Part model, mm, in its own coordinate system. A direction names the side the tool comes from. Coordinates: 2 decimals unless noted, no trailing zeros. Loops run counter-clockwise (first coordinate to the right, second up) from the corner with the lowest first, then second, coordinate; pieces in that order, holes last.
```python
from build123d import *

# Parameters (mm, degrees)
CROQUIS1_W              = 28
CROQUIS1_H              = 27.802688173
CROQUIS1_R              = 1.5
SALIENTE_EXTRUIR1_DEPTH = 3
CROQUIS2_W              = 3
CROQUIS2_H              = 12.401344086
CROQUIS2_H_2            = 3
CROQUIS2_H_3            = 12.401344087
CROQUIS2_W_2            = 12.5
SALIENTE_EXTRUIR2_DEPTH = 100
CROQUIS3_R              = 6.175
SALIENTE_EXTRUIR3_DEPTH = 13
CORTAR_EXTRUIR6_START   = 100
CROQUIS4_R              = 3.175
CORTAR_EXTRUIR6_DEPTH   = 10
CORTAR_EXTRUIR7_START   = 10.840894
CORTAR_EXTRUIR7_DEPTH   = 3
CORTAR_EXTRUIR8_START   = -31.5
CORTAR_EXTRUIR8_DEPTH   = 3
CROQUIS14_R             = 1.5
CORTAR_EXTRUIR9_DEPTH   = 12


with BuildPart() as part:
    # Croquis1 → Saliente-Extruir1 (new body)
    with BuildSketch(Plane.XY):
        with Locations((-33, 12.340894038)):
            Rectangle(CROQUIS1_W, CROQUIS1_H)
        with Locations((-39.5, 7)):
            Circle(CROQUIS1_R, mode=Mode.SUBTRACT)
        with Locations((-39.5, 21)):
            Circle(CROQUIS1_R, mode=Mode.SUBTRACT)
        with Locations((-25.5, 21)):
            Circle(CROQUIS1_R, mode=Mode.SUBTRACT)
        with Locations((-25.5, 7)):
            Circle(CROQUIS1_R, mode=Mode.SUBTRACT)
    extrude(amount=SALIENTE_EXTRUIR1_DEPTH)

    # Croquis2 → Saliente-Extruir2 (add)
    with BuildSketch(Plane.XY):
        with Locations((-33, 4.640221994)):
            Rectangle(CROQUIS2_W, CROQUIS2_H)
        with Locations((-33, 12.340894037)):
            Rectangle(CROQUIS2_W, CROQUIS2_H_2)
        with Locations((-33, 20.041566081)):
            Rectangle(CROQUIS2_W, CROQUIS2_H_3)
        with Locations((-25.25, 12.340894037)):
            Rectangle(CROQUIS2_W_2, CROQUIS2_H_2)
        with Locations((-40.75, 12.340894037)):
            Rectangle(CROQUIS2_W_2, CROQUIS2_H_2)
    extrude(amount=SALIENTE_EXTRUIR2_DEPTH)

    # Croquis3 → Saliente-Extruir3 (add)
    with BuildSketch(Plane.XY.offset(100)):
        with Locations((-33, 12.340894037)):
            Circle(CROQUIS3_R)
    extrude(amount=-SALIENTE_EXTRUIR3_DEPTH)

    # Croquis4 → Cortar-Extruir6 (cut)
    with BuildSketch(Plane.XY.offset(CORTAR_EXTRUIR6_START)):
        with Locations((-33, 12.340894037)):
            Circle(CROQUIS4_R)
    extrude(amount=-CORTAR_EXTRUIR6_DEPTH, mode=Mode.SUBTRACT)

    # Croquis12 → Cortar-Extruir7 (cut)
    with BuildSketch(Plane(origin=(0, 0, 0), x_dir=(1, 0, 0), z_dir=(0, 1, 0)).offset(CORTAR_EXTRUIR7_START)):
        Polygon((-47, -3), (-38.990043823, -87), (-38.990043823, -100), (-47, -100), align=None)
        Polygon((-19, -3), (-19, -100), (-27.009956177, -100), (-27.009956177, -87), align=None)
    extrude(amount=CORTAR_EXTRUIR7_DEPTH, mode=Mode.SUBTRACT)

    # Croquis13 → Cortar-Extruir8 (cut)
    with BuildSketch(Plane(origin=(0, 0, 0), x_dir=(0, 0, -1), z_dir=(1, 0, 0)).offset(CORTAR_EXTRUIR8_START)):
        Polygon((-100, 18.33093786), (-87, 18.33093786), (-3, 26.242238124), (-100, 26.242238124), align=None)
        Polygon((-100, -1.560450049), (-100, 6.350850214), (-87, 6.350850214), (-3, -1.560450049), align=None)
    extrude(amount=-CORTAR_EXTRUIR8_DEPTH, mode=Mode.SUBTRACT)

    # Croquis14 → Cortar-Extruir9 (cut)
    with BuildSketch(Plane.ZY.offset(38.990043823)):
        with Locations((93.5, 12.340894037)):
            Circle(CROQUIS14_R)
    extrude(amount=-CORTAR_EXTRUIR9_DEPTH, mode=Mode.SUBTRACT)


solid = part.part
```
Q1. Saw through at A-A (x = -25.5). List the corners of the cut face in (y, z), plus the area to 3 significant figures.
Q2. Probe line 1 (Y direction, x = -39.5, z = 1.15); line 2 (Z direction, x = -31.25, y = 14.5); line 3 (X direction, y = 21.25, z = 26). List the from-to ranges inside material, lowest first.
Q3. Tool access for faces 4 (the cylindrical face through (-37.4, 8.01, 93.59)), 5 (the flat face through (-27.01, 12, 98)), 6 (the flat face through (-36, 9, 87)): list every direction of +Z, -Z, +X, -X, +Y, -Y with a clear straight run to the whole face (end or side of a thin tool).
Q4. Mould opens along X. For faces 1 (the flat face through (-33, 18.331, 94)), 2 (the cylindrical face through (-28.67, 7.94, 93.59)), 3 (the flat face through (-33, 12, 90)) say: released by +X, released by -X, zero draft, split by the parting line, or undercut.
Q5. Saw through at D-D (z = 75). List the corners of the cut face in (x, y), plus the area to 3 significant figures.
Q6. Drop flat-ended pins along their axis: P1, Ø5, axis at x = -41, z = 81, coming from the +Y side; P2, Ø6, axis at x = -41, y = 6.5, coming from the +Z side; P3, Ø6, axis at y = 11.5, z = 31.5, coming from the +X side. Give the stop position or say it passes through.
Q7. Saw through at C-C (x = -33). List the corners of the cut face in (y, z), plus the area to 3 significant figures.
Q8. Saw through at B-B (y = 21). List the corners of the cut face in (x, z).
Checked values:
1. outline: (-1.56, 0) - (5.5, 0) - (5.5, 3) - (-1.56, 3) - close; (8.5, 0) - (19.5, 0) - (19.5, 3) - (13.84, 3) - (13.84, 71.17) - (10.84, 71.17) - (10.84, 3) - (8.5, 3) - close; (22.5, 0) - (26.24, 0) - (26.24, 3) - (22.5, 3) - close
1. area: 270 mm2
2. line 1: y = -1.56 to 5.5, 8.5 to 19.5, 22.5 to 26.24
2. line 2: z = 0 to 3, 87 to 90
2. line 3: x = -34.5 to -31.5
3. face 4: +Z, -X, -Y
3. face 5: +Z, +X, +Y, -Y
3. face 6: -X, -Y
4. face 1: zero draft
4. face 2: released by +X
4. face 3: undercut
5. outline: (-40.13, 10.84) - (-34.5, 10.84) - (-34.5, 5.22) - (-31.5, 5.22) - (-31.5, 10.84) - (-25.87, 10.84) - (-25.87, 13.84) - (-31.5, 13.84) - (-31.5, 19.46) - (-34.5, 19.46) - (-34.5, 13.84) - (-40.13, 13.84) - close
5. area: 76.5 mm2
6. P1: stops at y = 13.84
6. P2: stops at z = 3
6. P3: stops at x = -21.43
7. outline: (-1.56, 0) - (26.24, 0) - (26.24, 3) - (18.33, 87) - (18.33, 100) - (15.52, 100) - (15.52, 90) - (9.17, 90) - (9.17, 100) - (6.35, 100) - (6.35, 87) - (-1.56, 3) - close
7. area: 1,850 mm2
8. outline: (-47, 0) - (-41, 0) - (-41, 3) - (-47, 3) - close; (-38, 0) - (-27, 0) - (-27, 3) - (-31.5, 3) - (-31.5, 58.66) - (-34.5, 58.66) - (-34.5, 3) - (-38, 3) - close; (-24, 0) - (-19, 0) - (-19, 3) - (-24, 3) - close
